from build123d import *

# Parameters (mm, degrees)
SKETCH_1_W      = 120
SKETCH_1_H      = 15
SKETCH_1_R      = 5
EXTRUDE_2_DEPTH = 10
CHAMFER_2_SIZE  = 3


with BuildPart() as part:
    # 草图1 → 凸台-拉伸2 (new body)
    with BuildSketch(Plane.XY):
        with Locations((-12.990353698, 6.149517685)):
            Rectangle(SKETCH_1_W, SKETCH_1_H)
        with Locations((-64.990353698, 6.149517685)):
            Circle(SKETCH_1_R, mode=Mode.SUBTRACT)
        with Locations((39.009646302, 6.149517685)):
            Circle(SKETCH_1_R, mode=Mode.SUBTRACT)
        with Locations((-22.990353698, 6.149517685)):
            Circle(SKETCH_1_R, mode=Mode.SUBTRACT)
    extrude(amount=EXTRUDE_2_DEPTH)

    # 倒角2
    chamfer_2_edges = [part.edges().sort_by_distance(p)[0] for p in [
        (47.009646302, -1.350482315, 5),
        (-72.990353698, -1.350482315, 5),
        (-72.990353698, 13.649517685, 5),
        (47.009646302, 13.649517685, 5),
    ]]
    chamfer(chamfer_2_edges, length=CHAMFER_2_SIZE)


solid = part.part
Verification items for the finished model (mm, model axes). Give positions to 0.01 mm unless a question says otherwise; leave off trailing zeros. Order: outer loops, then holes, each group sorted by start corner. A loop starts at its lowest first (then second) coordinate and runs counter-clockwise, first axis right, second up. Notation, with made-up numbers: (68.25, -7.75) -> (126.25, -7.75) arc R14 ccw to (126.25, 16.25) -> close; hole circle Ø8 at (48, 77). An arc over 180 degrees is marked (long way). Answer as CSV lines item,"result".
Q1. Sectioned sample at B-B on x = -20.5. Record the cut outline in (y, z), plus the area to 3 significant figures.
Solutions:
outline,"(-1.35, 0) -> (1.81, 0) -> (1.81, 10) -> (-1.35, 10) -> close; (10.49, 0) -> (13.65, 0) -> (13.65, 10) -> (10.49, 10) -> close"
area,"63.3 mm²"
Q2. Release check for a two-part mould opening along Y. For faces 1 (the flat face through (-14, -1.35, 5)), 2 (the flat face through (-14, 13.65, 5)), 3 (the cylindrical face through (-27.986, 6.369, 4.93)) record: +Y half, -Y half, draft (parallel to the pull), parting line (faces both ways), or undercut.
Solutions:
face 1,"-Y half"
face 2,"+Y half"
face 3,"undercut"
Q3. Scan lines: probe 1 along X at (y, z) = (8.75, 7.25); probe 2 along X at (y, z) = (3, 3); probe 3 along Y at (x, z) = (-23.5, 8.5). Record each from-to range of solid material in increasing order.
Solutions:
probe 1,"x = -72.99 to -69.26, -60.72 to -27.26, -18.72 to 34.74, 43.28 to 47.01"
probe 2,"x = -72.99 to -68.87, -61.11 to -26.87, -19.11 to 35.13, 42.89 to 47.01"
probe 3,"y = -1.35 to 1.18, 11.12 to 13.65"
Q4. Sectioned sample at D-D on y = 12.25. Record the cut outline in (x, z).
Solutions:
outline,"(-71.39, 0) -> (45.41, 0) -> (45.41, 10) -> (-71.39, 10) -> close"
Q5. Sectioned sample at A-A on y = 7.5. Record the cut outline in (x, z).
Solutions:
outline,"(-72.99, 0) -> (-69.8, 0) -> (-69.8, 10) -> (-72.99, 10) -> close; (-60.18, 0) -> (-27.8, 0) -> (-27.8, 10) -> (-60.18, 10) -> close; (-18.18, 0) -> (34.2, 0) -> (34.2, 10) -> (-18.18, 10) -> close; (43.82, 0) -> (47.01, 0) -> (47.01, 10) -> (43.82, 10) -> close"
Q6. Sectioned sample at C-C on z = 7.25. Record the cut outline in (x, y), plus the area to 3 significant figures.
Solutions:
outline,"(-72.99, 1.65) -> (-69.99, -1.35) -> (44.01, -1.35) -> (47.01, 1.65) -> (47.01, 10.65) -> (44.01, 13.65) -> (-69.99, 13.65) -> (-72.99, 10.65) -> close; hole circle Ø10 at (-64.99, 6.15); hole circle Ø10 at (-22.99, 6.15); hole circle Ø10 at (39.01, 6.15)"
area,"1,550 mm²"
